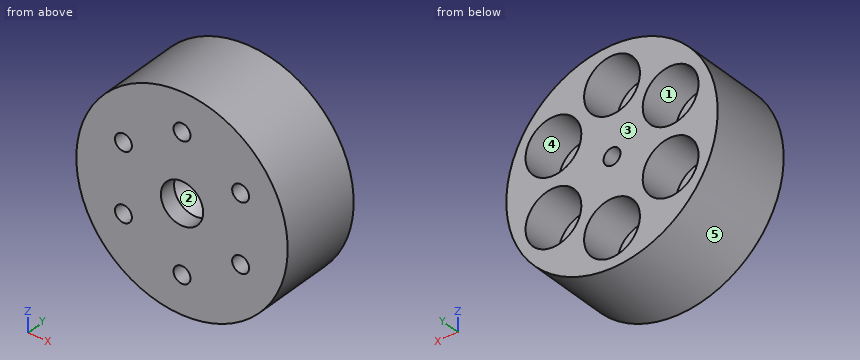
```python
from build123d import *

# Parameters (mm, degrees)
SKETCH1_R           = 25
BOSS_EXTRUDE1_DEPTH = 20
SKETCH2_R           = 6.6
CUT_EXTRUDE1_DEPTH  = 10
SKETCH3_R           = 2
CUT_EXTRUDE2_DEPTH  = 35
CIRPATTERN1_COUNT   = 6


with BuildPart() as part:
    # Sketch1 → Boss-Extrude1 (new body)
    with BuildSketch(Plane(origin=(0, 0, 0), x_dir=(1, 0, 0), z_dir=(0, 1, 0))):
        with Locations(Location((0, 0, 0), (0, 0, 270))):
            Circle(SKETCH1_R)
    extrude(amount=BOSS_EXTRUDE1_DEPTH)

    # Sketch2 → Cut-Extrude1 (cut)
    with BuildSketch(Plane(origin=(0, 20, 0), x_dir=(1, 0, 0), z_dir=(0, 1, 0))):
        with Locations(Location((0, 16, 0), (0, 0, 270))):
            Circle(SKETCH2_R)
    cut_extrude1 = extrude(amount=-CUT_EXTRUDE1_DEPTH, mode=Mode.SUBTRACT)

    # Sketch3 → Cut-Extrude2 (cut)
    with BuildSketch(Plane(origin=(0, 10, 0), x_dir=(1, 0, 0), z_dir=(0, 1, 0))):
        with Locations(Location((0, 16, 0), (0, 0, 270))):
            Circle(SKETCH3_R)
    cut_extrude2 = extrude(amount=-CUT_EXTRUDE2_DEPTH, mode=Mode.SUBTRACT)

    # CirPattern1: Cut-Extrude1, Cut-Extrude2 ×6 about axis
    cirpattern1_axis = Axis((0, 0, 0), (0, 1, 0))
    add([cut_extrude1.rotate(cirpattern1_axis, i * 360 / CIRPATTERN1_COUNT) for i in range(1, CIRPATTERN1_COUNT)], mode=Mode.SUBTRACT)
    add([cut_extrude2.rotate(cirpattern1_axis, i * 360 / CIRPATTERN1_COUNT) for i in range(1, CIRPATTERN1_COUNT)], mode=Mode.SUBTRACT)

    # Sketch5 → Cut-Revolve1 (revolve, cut)
    with BuildSketch(Plane.XY, mode=Mode.PRIVATE) as cut_revolve1_sk:
        Polygon((0, 20), (-2, 20), (-2, 7), (-5, 4), (-5, 0), (0, 0), align=None)
    revolve(cut_revolve1_sk.sketch.rotate(Axis((0, 26.035493364, 0), (0, -1, 0)), 270), axis=Axis((0, 26.035493364, 0), (0, -1, 0)), mode=Mode.SUBTRACT)


solid = part.part
```
Geometry check sheet. Reference: the model listing, model coordinates, mm. Face numbers are marked on the shaded views. A direction names the side the tool comes from. Coordinates: 2 decimals unless noted, no trailing zeros. Loops run counter-clockwise (first coordinate to the right, second up) from the corner with the lowest first, then second, coordinate; pieces in that order, holes last. Notation, with made-up numbers: (-8.5, 30) - (46.5, 30) arc R27 ccw to (46.5, 68) - close; hole circle Ø5 at (-32, 39.5). An arc over 180 degrees is marked (long way). One line per item, written item: value. Start each with the question number.
(1) Tool access check on the marked faces 1 and 2. Record the directions out of +Z, -Z, +X, -X, +Y, -Y that give a thin tool (end or side, any length) a straight path to the whole face; none if there is none.
(2) Depth check by flat-ended pin: P1, Ø5, axis at x = 16.5, y = 12, coming from the -Z side; P2, Ø2, axis at x = -16, z = -6.5, coming from the +Y side; P3, Ø1.5, axis at x = -19.5, y = 2.5, coming from the -Z side. Enter the tip coordinate at first touch or a pass-through.
(3) Cross-section at C-C on y = 16. Enter the section's corners in (x, z), plus the area to 3 significant figures.
(4) Mould release check, pull along Z, two halves, no side actions. Record for the marked faces 3, 4 and 5: released by +Z, released by -Z, zero draft, split by the parting line, or undercut.
(5) Cross-section at D-D on z = 8. Enter the section's corners in (x, y).
(6) Cross-section at B-B on x = 0. Enter the section's corners in (y, z), plus the area to 3 significant figures.
(7) Cross-section at A-A on z = 0. Enter the section's corners in (x, y).
(8) Material ranges on line 1 (X direction, y = 16.25, z = 0); line 2 (X direction, y = 4, z = 8); line 3 (Z direction, x = -0.5, y = 5.75) (1 decimal), recorded low to high. Write a range as [from, to].
Results below:
1. face 1: +Y
1. face 2: -Y
2. P1: stops at z = -20.71
2. P2: stops at y = 10
2. P3: stops at z = -16.54
3. outline: circle Ø50 at (0, 0); hole circle Ø13.2 at (-13.86, -8); hole circle Ø13.2 at (-13.86, 8); hole circle Ø13.2 at (0, -16); hole circle Ø13.2 at (0, 16); hole circle Ø4 at (0, 0); hole circle Ø13.2 at (13.86, -8); hole circle Ø13.2 at (13.86, 8)
3. area: 1,130 mm2
4. face 3: zero draft
4. face 4: undercut
4. face 5: split by the parting line
5. outline: (-23.69, 0) - (-15.86, 0) - (-15.86, 10) - (-20.46, 10) - (-20.46, 20) - (-23.69, 20) - close; (-11.86, 0) - (11.86, 0) - (11.86, 10) - (7.26, 10) - (7.26, 20) - (-7.26, 20) - (-7.26, 10) - (-11.86, 10) - close; (15.86, 0) - (23.69, 0) - (23.69, 20) - (20.46, 20) - (20.46, 10) - (15.86, 10) - close
6. outline: (0, -25) - (20, -25) - (20, -22.6) - (10, -22.6) - (10, -18) - (0, -18) - close; (0, -14) - (10, -14) - (10, -9.4) - (20, -9.4) - (20, -2) - (7, -2) - (4, -5) - (0, -5) - close; (0, 5) - (4, 5) - (7, 2) - (20, 2) - (20, 9.4) - (10, 9.4) - (10, 14) - (0, 14) - close; (0, 18) - (10, 18) - (10, 22.6) - (20, 22.6) - (20, 25) - (0, 25) - close
6. area: 543 mm2
7. outline: (-25, 0) - (-5, 0) - (-5, 4) - (-2, 7) - (-2, 20) - (-25, 20) - close; (2, 7) - (5, 4) - (5, 0) - (25, 0) - (25, 20) - (2, 20) - close
8. line 1: x = [-25, -2], [2, 25]
8. line 2: x = [-23.69, -15.86], [-11.86, 11.86], [15.86, 23.69]
8. line 3: z = [-25, -17.9], [-14.1, -3.2], [3.2, 14.1], [17.9, 25]
